Verification items for this drawing (mm, ordinates from the low corner). Coordinates: 2 decimals unless noted, no trailing zeros. Write each loop counter-clockwise with the first axis right and the second up, starting at its lowest first coordinate (ties: lowest second). Pieces come first, ordered by that corner, then holes.
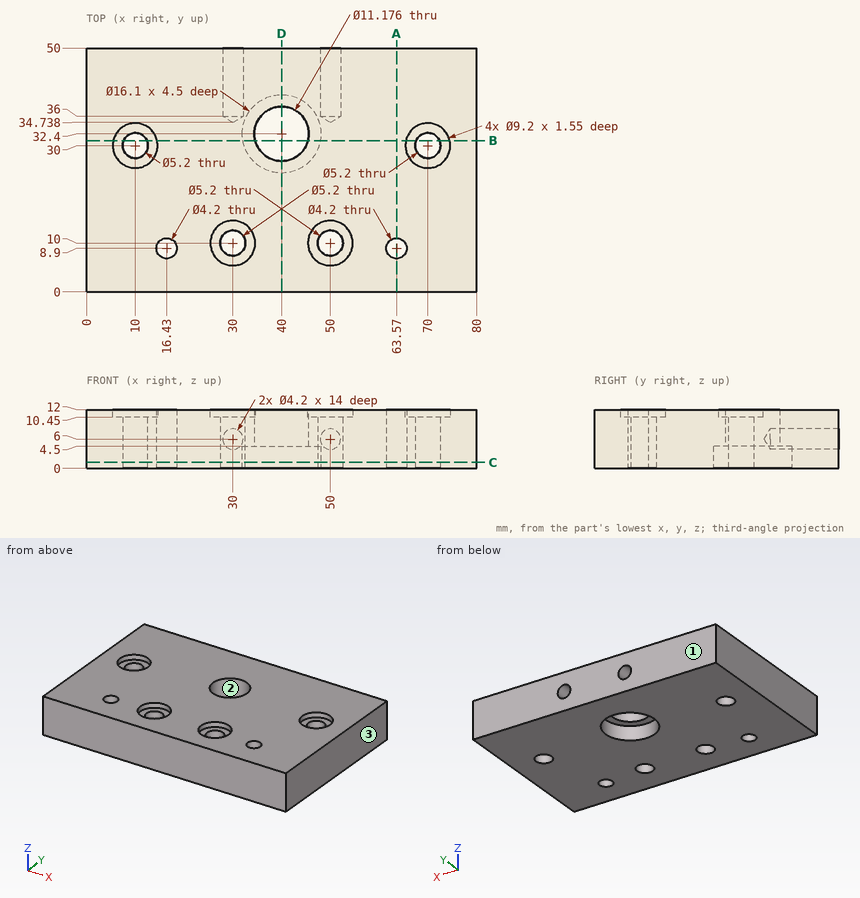
1. Sectioned sample at B-B, the plane y = 31. Record the boundary of the cut face in (x, z), and give its area (3 significant figures).
Computed values:
outline: (0, 0) - (7.6, 0) - (7.6, 10.45) - (5.51, 10.45) - (5.51, 12) - (0, 12) - close; (12.4, 0) - (32.07, 0) - (32.07, 4.5) - (34.59, 4.5) - (34.59, 12) - (14.49, 12) - (14.49, 10.45) - (12.4, 10.45) - close; (45.41, 4.5) - (47.93, 4.5) - (47.93, 0) - (67.6, 0) - (67.6, 10.45) - (65.51, 10.45) - (65.51, 12) - (45.41, 12) - close; (72.4, 0) - (80, 0) - (80, 12) - (74.49, 12) - (74.49, 10.45) - (72.4, 10.45) - close
area: 679 mm2
2. Gauge pin test, flat ends, axial feed: pin 1 Ø2 at (x, y) = (42.5, 38) entering from -Z; pin 2 Ø4.5 at (x, y) = (29, 8.5) entering from +Z; pin 3 Ø2.5 at (x, z) = (30, 6) entering from +Y. Record the tip position at first contact, or that the pin passes through.
Computed values:
pin 1: stops at z = 4.5
pin 2: stops at z = 10.45
pin 3: stops at y = 35.49
3. Draft check along X on the marked faces 1, 2 and 3. Enter one of: released by +X, released by -X, zero draft, split by the parting line, or undercut.
Computed values:
face 1: zero draft
face 2: undercut
face 3: released by +X
4. Thickness scan on line 1 along Y through (x, z) = (10, 10.85); line 2 along X through (y, z) = (10.5, 1.25); line 3 along Y through (x, z) = (70, 4.75). Record the ranges inside material, lowest first.
Computed values:
line 1: y = 0 to 25.4, 34.6 to 50
line 2: x = 0 to 15.07, 17.79 to 27.45, 32.55 to 47.45, 52.55 to 62.21, 64.93 to 80
line 3: y = 0 to 27.4, 32.6 to 50
5. Sectioned sample at A-A, the plane x = 63.57. Record the boundary of the cut face in (y, z), and give its area (3 significant figures).
Computed values:
outline: (0, 0) - (6.8, 0) - (6.8, 12) - (0, 12) - close; (11, 0) - (50, 0) - (50, 12) - (11, 12) - close
area: 550 mm2
6. Sectioned sample at C-C, the plane z = 1.25. Record the boundary of the cut face in (x, y).
Computed values:
outline: (0, 0) - (80, 0) - (80, 50) - (0, 50) - close; hole circle Ø5.2 at (10, 30); hole circle Ø4.2 at (16.43, 8.9); hole circle Ø5.2 at (30, 10); hole circle Ø16.1 at (40, 32.4); hole circle Ø5.2 at (50, 10); hole circle Ø4.2 at (63.57, 8.9); hole circle Ø5.2 at (70, 30)
7. Sectioned sample at D-D, the plane x = 40. Record the boundary of the cut face in (y, z), and give its area (3 significant figures).
Computed values:
outline: (0, 0) - (24.35, 0) - (24.35, 4.5) - (26.81, 4.5) - (26.81, 12) - (0, 12) - close; (37.99, 4.5) - (40.45, 4.5) - (40.45, 0) - (50, 0) - (50, 12) - (37.99, 12) - close
area: 444 mm2
